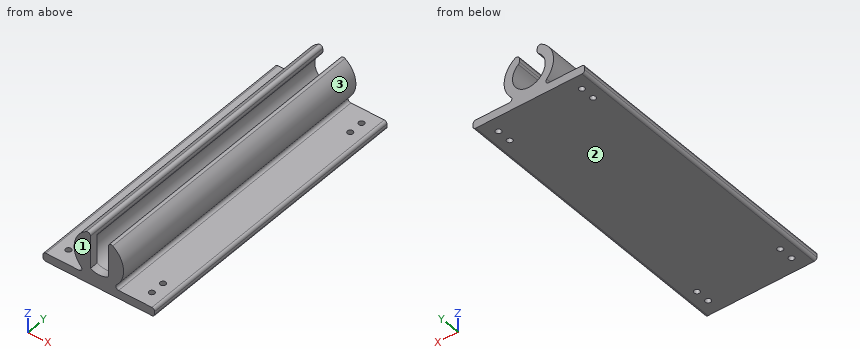
from build123d import *

# Parameters (mm, degrees)
F1_DEPTH = 101.6
F3_DEPTH = 3
F4_R     = 1
F5_DEPTH = 25.4
F6_R     = 1
F7_R     = 1


with BuildPart() as f1:
    # F0 (on Front) → F1 (new body)
    with BuildSketch(Plane.XZ):
        with BuildLine():
            ThreePointArc((3.4161663997, 4.7504878758), (-0.2489109402, -5.8459705159), (-3, 5.0236767341))
            Line((-3, 5.0236767341), (-3, 8.3273603964))
            ThreePointArc((-3, 8.3273603964), (-8.83136125, 0.5932871507), (-4.0868734277, -7.8512672071))
            Line((-4.0868734277, -7.8512672071), (-20, -7.8512672071))
            Line((-20, -7.8512672071), (-20, -10.8512672071))
            Line((-20, -10.8512672071), (20, -10.8512672071))
            Line((20, -10.8512672071), (20, -7.8512672071))
            Line((20, -7.8512672071), (4.0868734277, -7.8512672071))
            ThreePointArc((4.0868734277, -7.8512672071), (8.8435168288, 0.3703258964), (3.4161663997, 8.165460079))
            Line((3.4161663997, 8.165460079), (3.4161663997, 4.7504878758))
        make_face()
    extrude(amount=F1_DEPTH)

    # F2 (on face) → F3 (join)
    with BuildSketch(Plane.XZ.offset(101.6)):
        with BuildLine():
            Line((-3, -5.0236767341), (-3, 8.3273603964))
            ThreePointArc((-3, 8.3273603964), (-8.83136125, 0.5932871507), (-4.0868734277, -7.8512672071))
            Line((-4.0868734277, -7.8512672071), (-20, -7.8512672071))
            Line((-20, -7.8512672071), (-20, -10.8512672071))
            Line((-20, -10.8512672071), (20, -10.8512672071))
            Line((20, -10.8512672071), (20, -7.8512672071))
            Line((20, -7.8512672071), (4.0868734277, -7.8512672071))
            ThreePointArc((4.0868734277, -7.8512672071), (8.8435168288, 0.3703258964), (3.4161663997, 8.165460079))
            Line((3.4161663997, 8.165460079), (3.4161663997, -4.7504878758))
            ThreePointArc((3.4161663997, -4.7504878758), (0.2489109402, -5.8459705159), (-3, -5.0236767341))
        make_face()
    extrude(amount=F3_DEPTH)

    # F4 (on Top) → F5 (cut)
    with BuildSketch(Plane.XY):
        with Locations((-14.92, -5.08)):
            Circle(F4_R)
        with Locations((-14.92, -10.16)):
            Circle(F4_R)
        with Locations((-14.92, -99.52)):
            Circle(F4_R)
        with Locations((-14.92, -94.44)):
            Circle(F4_R)
        with Locations((14.92, -99.52)):
            Circle(F4_R)
        with Locations((14.92, -94.44)):
            Circle(F4_R)
        with Locations((14.92, -10.16)):
            Circle(F4_R)
        with Locations((14.92, -5.08)):
            Circle(F4_R)
    extrude(amount=-F5_DEPTH, mode=Mode.SUBTRACT)

    # F6
    f6_edges = [f1.edges().sort_by_distance(p)[0] for p in [
        (-3, -52.3, 8.32736),
        (3.416166, -52.3, 8.16546),
        (-3, -50.8, 5.023677),
        (3.416166, -50.8, 4.750488),
    ]]
    fillet(f6_edges, radius=F6_R)

    # F7
    f7_edges = [f1.edges().sort_by_distance(p)[0] for p in [
        (20, -52.3, -7.851267),
        (20, -52.3, -10.851267),
        (-20, -52.3, -7.851267),
        (-20, -52.3, -10.851267),
        (4.086873, -52.3, -7.851267),
        (-4.086873, -52.3, -7.851267),
    ]]
    fillet(f7_edges, radius=F7_R)


solid = f1.part
Geometry check sheet. Reference: the model listing, model coordinates, mm. Face numbers are marked on the shaded views. Round coordinates to 2 decimals unless told otherwise and drop trailing zeros. Loops run counter-clockwise (first coordinate to the right, second up) from the corner with the lowest first, then second, coordinate; pieces in that order, holes last. Notation, with made-up numbers: (1.5, 44) - (18.5, 44) arc R15 cw to (18.5, 72) - close; hole circle Ø10 at (-8, 82.25). An arc over 180 degrees is marked (long way). One line per question, with ' | ' between items. Start each with the question number.
1. Depth check by flat-ended pin: pin 1 (1.6 mm diameter, centred on x = -14.92, y = -10.16, fed in from +Z); pin 2 (1.5 mm diameter, centred on x = 12.5, y = -11, fed in from +Z); pin 3 (2 mm diameter, centred on y = -20.5, z = -1.5, fed in from -X); pin 4 (2.5 mm diameter, centred on x = -14.92, y = -94.44, fed in from -Z). Enter the tip coordinate at first touch or a pass-through.
2. Scan lines: line 1 (Y direction, x = -14.92, z = -8.7); line 2 (X direction, y = -59, z = 0); line 3 (X direction, y = -99.52, z = -9.55). Record each from-to range of solid material in increasing order. Write a range as [from, to].
3. Cross-section at B-B on x = -14.92. Record the cut outline in (y, z), then the cut area to 3 significant figures.
4. Cross-section at C-C on y = -99.52. Record the cut outline in (x, z), then the cut area to 3 significant figures.
5. Draft check along Z on the marked faces 1, 2 and 3. Enter one of: released by +Z, released by -Z, zero draft, split by the parting line, or undercut.
6. Cross-section at D-D on y = -46.5. Record the cut outline in (x, z).
7. Cross-section at A-A on z = 0. Record the cut outline in (x, y), then the cut area to 3 significant figures.
Taken from the geometry:
1) pin 1: through | pin 2: z = -7.85 | pin 3: x = -8.84 | pin 4: z = -10.85
2) line 1: [-104.6, -100.52], [-98.52, -95.44], [-93.44, -11.16], [-9.16, -6.08], [-4.08, 0] | line 2: [-8.85, -5.85], [5.85, 8.85] | line 3: [-20, -15.92], [-13.92, 13.92], [15.92, 20]
3) outline: (-104.6, -10.85) - (-100.52, -10.85) - (-100.52, -7.85) - (-104.6, -7.85) - close; (-98.52, -10.85) - (-95.44, -10.85) - (-95.44, -7.85) - (-98.52, -7.85) - close; (-93.44, -10.85) - (-11.16, -10.85) - (-11.16, -7.85) - (-93.44, -7.85) - close; (-9.16, -10.85) - (-6.08, -10.85) - (-6.08, -7.85) - (-9.16, -7.85) - close; (-4.08, -10.85) - (0, -10.85) - (0, -7.85) - (-4.08, -7.85) - close | area: 290 mm²
4) outline: (-20, -9.85) arc R1 ccw to (-19, -10.85) - (-15.92, -10.85) - (-15.92, -7.85) - (-19, -7.85) arc R1 ccw to (-20, -8.85) - close; (-13.92, -10.85) - (13.92, -10.85) - (13.92, -7.85) - (7.08, -7.85) arc R1 cw to (6.36, -6.16) arc R8.85 ccw to (4.98, 7.32) arc R1 ccw to (3.42, 6.49) - (3.42, 5.24) arc R1 ccw to (3.77, 4.47) arc R5.85 cw (long way) to (-3.42, 4.75) arc R1 ccw to (-3, 5.56) - (-3, 6.76) arc R1 ccw to (-4.51, 7.62) arc R8.85 ccw to (-6.36, -6.16) arc R1 cw to (-7.08, -7.85) - (-13.92, -7.85) - close; (15.92, -10.85) - (19, -10.85) arc R1 ccw to (20, -9.85) - (20, -8.85) arc R1 ccw to (19, -7.85) - (15.92, -7.85) - close | area: 222 mm²
5) face 1: zero draft | face 2: released by -Z | face 3: undercut
6) outline: (-20, -9.85) arc R1 ccw to (-19, -10.85) - (19, -10.85) arc R1 ccw to (20, -9.85) - (20, -8.85) arc R1 ccw to (19, -7.85) - (7.08, -7.85) arc R1 cw to (6.36, -6.16) arc R8.85 ccw to (4.98, 7.32) arc R1 ccw to (3.42, 6.49) - (3.42, 5.24) arc R1 ccw to (3.77, 4.47) arc R5.85 cw (long way) to (-3.42, 4.75) arc R1 ccw to (-3, 5.56) - (-3, 6.76) arc R1 ccw to (-4.51, 7.62) arc R8.85 ccw to (-6.36, -6.16) arc R1 cw to (-7.08, -7.85) - (-19, -7.85) arc R1 ccw to (-20, -8.85) - close
7) outline: (-8.85, -104.6) - (-3, -104.6) - (-3, -101.6) - (-5.85, -101.6) - (-5.85, 0) - (-8.85, 0) - close; (3.42, -104.6) - (8.85, -104.6) - (8.85, 0) - (5.85, 0) - (5.85, -101.6) - (3.42, -101.6) - close | area: 643 mm²
